```python
from build123d import *

# Parameters (mm, degrees)
SKETCH_W        = 40
SKETCH_H        = 30
PAD_DEPTH       = 2
SKETCH001_W     = 33.6
SKETCH001_H     = 24.9
PAD001_DEPTH    = 1
SKETCH002_R     = 1
POCKET_DEPTH    = 2
FILLET_R        = 0.5
SKETCH003_R     = 1
POCKET001_DEPTH = 2


with BuildPart() as part:
    # Sketch → Pad (new body)
    with BuildSketch(Plane.XY.offset(2)):
        Rectangle(SKETCH_W, SKETCH_H)
    extrude(amount=PAD_DEPTH)

    # Sketch001 (on Face6 of Pad) → Pad001 (join)
    with BuildSketch(Plane.XY.offset(4)):
        Rectangle(SKETCH001_W, SKETCH001_H)
    extrude(amount=PAD001_DEPTH)

    # Sketch002 → Pocket (cut)
    with BuildSketch(Plane.XY.offset(2)):
        with Locations((-18.4, 13.75)):
            Circle(SKETCH002_R)
        with Locations((-6.4, 13.75)):
            Circle(SKETCH002_R)
        with Locations((6.4, 13.75)):
            Circle(SKETCH002_R)
        with Locations((18.4, 13.75)):
            Circle(SKETCH002_R)
        with Locations((18.4, -13.75)):
            Circle(SKETCH002_R)
        with Locations((6.4, -13.75)):
            Circle(SKETCH002_R)
        with Locations((-6.4, -13.75)):
            Circle(SKETCH002_R)
        with Locations((-18.4, -13.75)):
            Circle(SKETCH002_R)
    extrude(amount=POCKET_DEPTH, mode=Mode.SUBTRACT)

    # Fillet
    fillet_edges = [part.edges().sort_by_distance(p)[0] for p in [
        (20, 15, 3),
        (16.8, 12.45, 4.5),
        (20, -15, 3),
        (16.8, -12.45, 4.5),
        (-20, -15, 3),
        (-16.8, -12.45, 4.5),
        (-20, 15, 3),
        (-16.8, 12.45, 4.5),
    ]]
    fillet(fillet_edges, radius=FILLET_R)

    # Sketch003 (on Face2 of Fillet) → Pocket001 (cut)
    with BuildSketch(Plane(origin=(0, 0, 2), x_dir=(1, 0, 0), z_dir=(0, 0, -1))):
        with Locations((-10, 5)):
            Circle(SKETCH003_R)
        with Locations((0, 5)):
            Circle(SKETCH003_R)
        with Locations((10, 5)):
            Circle(SKETCH003_R)
        with Locations((-10, -5)):
            Circle(SKETCH003_R)
        with Locations((0, -5)):
            Circle(SKETCH003_R)
        with Locations((10, -5)):
            Circle(SKETCH003_R)
    extrude(amount=-POCKET001_DEPTH, mode=Mode.SUBTRACT)


solid = part.part
```
Can you work these out from the model? Positions are in its coordinate system, mm. A direction names the side the tool comes from. Round coordinates to 2 decimals unless told otherwise and drop trailing zeros. Loops run counter-clockwise (first coordinate to the right, second up) from the corner with the lowest first, then second, coordinate; pieces in that order, holes last. Notation, with made-up numbers: (42, -34.75) -> (80, -34.75) arc R19 ccw to (80, -20.75) -> close; hole circle Ø4 at (-29, 11.5). An arc over 180 degrees is marked (long way). Answer in a Markdown table with one row per item.
Item 1: Will these pins go through, and if not, where does the flat tip stop? P1, Ø0.6, axis at x = 10, y = -5.5, coming from the -Z side; P2, Ø0.8, axis at x = -2, z = 4.5, coming from the +Y side.
Answer block:
| item | result |
|---|---|
| P1 | z = 4 |
| P2 | y = 12.45 |
Item 2: Suppose I cut it at B-B, the plane x = 6.4. List the corners of the cut face in (y, z) for me, plus the area to 3 significant figures.
Answer block:
| item | result |
|---|---|
| outline | (-15, 2) -> (-14.75, 2) -> (-14.75, 4) -> (-15, 4) -> close; (-12.75, 2) -> (12.75, 2) -> (12.75, 4) -> (12.45, 4) -> (12.45, 5) -> (-12.45, 5) -> (-12.45, 4) -> (-12.75, 4) -> close; (14.75, 2) -> (15, 2) -> (15, 4) -> (14.75, 4) -> close |
| area | 76.9 mm² |
Item 3: Suppose I cut it at C-C, the plane z = 3.5. Give the number of separate pieces and of enclosed holes in the cut face, plus the area to 3 significant figures.
Answer block:
| item | result |
|---|---|
| separate pieces | 1 |
| enclosed holes | 14 |
| area | 1,160 mm² |
Item 4: Suppose I cut it at D-D, the plane y = -5. List the corners of the cut face in (x, z) for me.
Answer block:
| item | result |
|---|---|
| outline | (-20, 2) -> (-11, 2) -> (-11, 4) -> (-9, 4) -> (-9, 2) -> (-1, 2) -> (-1, 4) -> (1, 4) -> (1, 2) -> (9, 2) -> (9, 4) -> (11, 4) -> (11, 2) -> (20, 2) -> (20, 4) -> (16.8, 4) -> (16.8, 5) -> (-16.8, 5) -> (-16.8, 4) -> (-20, 4) -> close |
Item 5: We'd pull the mould along X, two halves only. Please class faces 5 (the cylindrical face through (0, -6, 3)), 6 (the flat face through (20, 0, 3)), 7 (the flat face through (0, 15, 3)): released by +X, released by -X, zero draft, split by the parting line, or undercut.
Answer block:
| item | result |
|---|---|
| face 5 | undercut |
| face 6 | released by +X |
| face 7 | zero draft |
Item 6: Suppose I cut it at A-A, the plane y = 13.75. List the corners of the cut face in (x, z) for me.
Answer block:
| item | result |
|---|---|
| outline | (-20, 2) -> (-19.4, 2) -> (-19.4, 4) -> (-20, 4) -> close; (-17.4, 2) -> (-7.4, 2) -> (-7.4, 4) -> (-17.4, 4) -> close; (-5.4, 2) -> (5.4, 2) -> (5.4, 4) -> (-5.4, 4) -> close; (7.4, 2) -> (17.4, 2) -> (17.4, 4) -> (7.4, 4) -> close; (19.4, 2) -> (20, 2) -> (20, 4) -> (19.4, 4) -> close |
Item 7: On a 3-axis mill with a long thin cutter (end or side, diameter ignored), from which of +Z, -Z, +X, -X, +Y, -Y can I reach the whole of each face in a straight line? I mean faces 1 (the cylindrical face through (18.86, -14.64, 2.99)), 2 (the flat face through (-0.2, -12.45, 4.5)), 3 (the flat face through (0, -13, 4)), 4 (the cylindrical face through (9.263, 4.324, 2.986)). Say none if no direction works.
Answer block:
| item | result |
|---|---|
| face 1 | +Z, -Z |
| face 2 | +Z, +X, -X, -Y |
| face 3 | +Z |
| face 4 | -Z |
Item 8: If I drill on probe 1 along Y at (x, z) = (-10, 3.5); probe 2 along Y at (x, z) = (6.4, 2.5); probe 3 along X at (y, z) = (-5, 3.5), over which ranges is the centre line in solid material (lowest first)?
Answer block:
| item | result |
|---|---|
| probe 1 | -15 to -6, -4 to 4, 6 to 15 |
| probe 2 | -15 to -14.75, -12.75 to 12.75, 14.75 to 15 |
| probe 3 | -20 to -11, -9 to -1, 1 to 9, 11 to 20 |
